```python
from build123d import *

# Parameters (mm, degrees)
F1_DEPTH = 22.098
F2_DEPTH = 12.7
F3_DEPTH = 10.16
F4_DEPTH = 17.78
F5_DEPTH = 25.4


with BuildPart() as f1:
    # F0 (on Top) → F1 (new body)
    with BuildSketch(Plane.XY):
        Polygon((-4.405003, 8.097968), (-4.405003, 15.717968), (-17.105003, 15.717968), (-17.105003, 3.017968), (-9.622183, 3.017968), (-9.485003, 3.017968), (-9.485003, 8.097968), align=None)
    extrude(amount=F1_DEPTH)

    # F0 (on Top) → F2 (join)
    with BuildSketch(Plane.XY):
        Polygon((0.674997, 3.017968), (8.294997, 3.017968), (8.294997, 15.717968), (-4.405003, 15.717968), (-4.405003, 8.097968), (0.674997, 8.097968), align=None)
    extrude(amount=F2_DEPTH)

    # F0 (on Top) → F3 (join)
    with BuildSketch(Plane.XY):
        Polygon((-17.105003, -9.682032), (-4.405003, -9.682032), (-4.405003, -2.062032), (-9.485003, -2.062032), (-9.485003, 3.017968), (-9.622183, 3.017968), (-17.105003, 3.017968), (-17.105003, -3.333643), align=None)
    extrude(amount=F3_DEPTH)

    # F0 (on Top) → F4 (join)
    with BuildSketch(Plane.XY):
        Polygon((-4.405003, -9.682032), (8.294997, -9.682032), (8.294997, 3.017968), (0.674997, 3.017968), (0.674997, -2.062032), (-4.405003, -2.062032), align=None)
    extrude(amount=F4_DEPTH)

    # F0 (on Top) → F5 (join)
    with BuildSketch(Plane.XY):
        Polygon((-9.485003, -2.062032), (-4.405003, -2.062032), (0.674997, -2.062032), (0.674997, 3.017968), (0.674997, 8.097968), (-4.405003, 8.097968), (-9.485003, 8.097968), (-9.485003, 3.017968), align=None)
    extrude(amount=F5_DEPTH)


solid = f1.part
```
CAD build for the part. Positions are in the model's coordinates, mm. A direction names the side the tool comes from. Round coordinates to 2 decimals unless told otherwise and drop trailing zeros. Write each loop counter-clockwise with the first axis right and the second up, starting at its lowest first coordinate (ties: lowest second). Pieces come first, ordered by that corner, then holes. Notation, with made-up numbers: (54, -23) - (92, -23) arc R14 ccw to (92, -8) - close; hole circle Ø11 at (82, 81). An arc over 180 degrees is marked (long way). Return JSON: item names as keys, results as strings. Group by question number.
Item 1: Band-saw the part on A-A on z = 15.25. List the corners of the cut face in (x, y) (3 decimals).
Item 2: Band-saw the part on B-B on x = -13. List the corners of the cut face in (y, z).
Item 3: Probe probe 1 along Z at (x, y) = (0.75, -5.75); probe 2 along Z at (x, y) = (1.25, 4.25); probe 3 along Y at (x, z) = (-3.5, 14.25). List the from-to ranges inside material, lowest first.
Item 4: Band-saw the part on D-D on z = 21. List the corners of the cut face in (x, y) (3 decimals).
Item 5: Flat gauge pins, fed straight in: pin 1 Ø6 at (y, z) = (12, 18) entering from +X (3 decimals); pin 2 Ø3 at (x, y) = (0.5, -6) entering from +Z; pin 3 Ø1.5 at (x, z) = (5, 14) entering from +Y. Where does each tip first touch, or does it go through?
Item 6: 3-axis set-ups, long thin cutter, end or side, ignore diameter. For faces 1 (the face through (-4.405, 12, 17)), 2 (the face through (-4.405, -6, 14)), 3 (the face through (-5, 3, 0)): which of +Z, -Z, +X, -X, +Y, -Y reach the whole face in a straight line?
Item 7: Band-saw the part on C-C on y = -0.5. List the corners of the cut face in (x, z) (3 decimals).
Resolved:
{
 "1": {"outline": "(-17.105, 3.018) - (-9.485, 3.018) - (-9.485, -2.062) - (-4.405, -2.062) - (-4.405, -9.682) - (8.295, -9.682) - (8.295, 3.018) - (0.675, 3.018) - (0.675, 8.098) - (-4.405, 8.098) - (-4.405, 15.718) - (-17.105, 15.718) - close"},
 "2": {"outline": "(-9.68, 0) - (15.72, 0) - (15.72, 22.1) - (3.02, 22.1) - (3.02, 10.16) - (-9.68, 10.16) - close"},
 "3": {"probe 1": "z = 0 to 17.78", "probe 2": "z = 0 to 12.7", "probe 3": "y = -9.68 to 8.1"},
 "4": {"outline": "(-17.105, 3.018) - (-9.485, 3.018) - (-9.485, -2.062) - (0.675, -2.062) - (0.675, 8.098) - (-4.405, 8.098) - (-4.405, 15.718) - (-17.105, 15.718) - close"},
 "5": {"pin 1": "stops at x = -4.405", "pin 2": "stops at z = 17.78", "pin 3": "stops at y = 3.02"},
 "6": {"face 1": "+Z, +X, +Y", "face 2": "+Z, -X, -Y", "face 3": "-Z, +X, -X, +Y, -Y"},
 "7": {"outline": "(-17.105, 0) - (8.295, 0) - (8.295, 17.78) - (0.675, 17.78) - (0.675, 25.4) - (-9.485, 25.4) - (-9.485, 10.16) - (-17.105, 10.16) - close"}
}
